Source: three-view drawing plus pictorial views. Frame: mm from the lowest corner of the part. Coordinates: 2 decimals unless noted, no trailing zeros. Write each loop counter-clockwise with the first axis right and the second up, starting at its lowest first coordinate (ties: lowest second). Pieces come first, ordered by that corner, then holes. Notation, with made-up numbers: (77.5, 53.25) - (98.5, 53.25) arc R37 ccw to (98.5, 92.25) - close; hole circle Ø9 at (39, 8). An arc over 180 degrees is marked (long way). One line per item, written item: value.
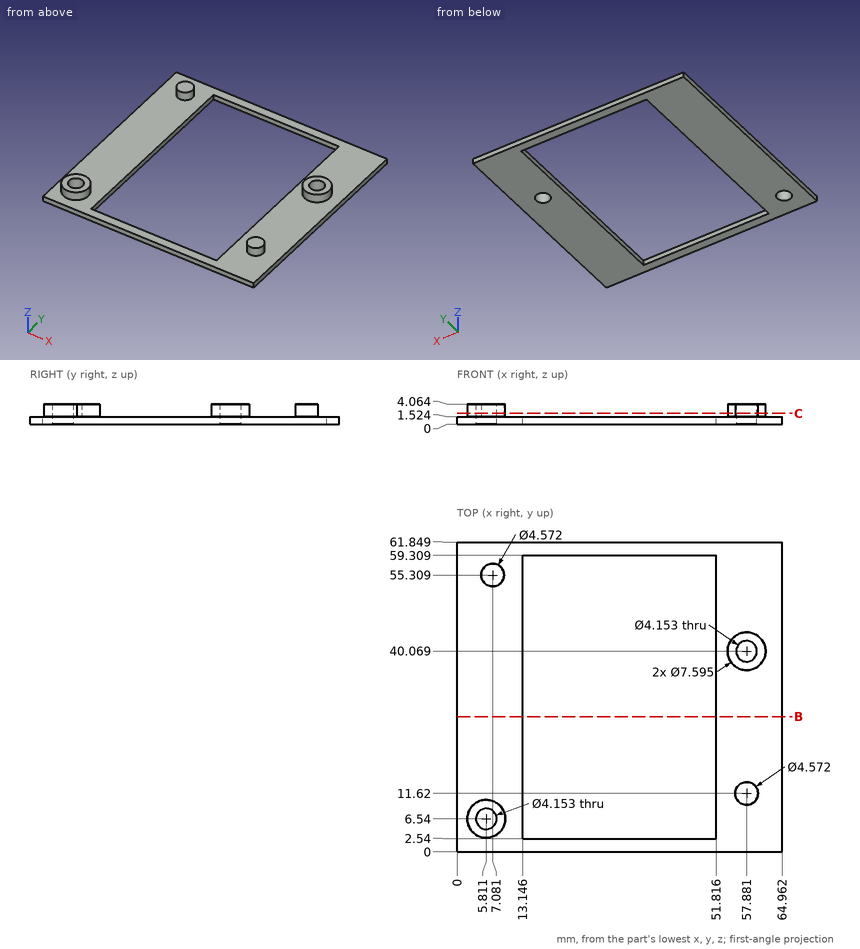
1) Section query C-C on z = 2.2. Output: boundary loops of the cut face in (x, y) (1 decimal).
Values found:
outline: circle Ø7.6 at (5.8, 6.5); circle Ø4.6 at (7.1, 55.3); circle Ø7.6 at (57.9, 40.1); circle Ø4.6 at (57.9, 11.6); hole circle Ø4.2 at (5.8, 6.5); hole circle Ø4.2 at (57.9, 40.1)
2) Contact query for a flat-ended pin moving along its axis: P1, Ø10, axis at x = 7, y = 33, coming from the +Z side. Output: stop coordinate, or through.
Values found:
P1: z = 1.52
3) Material intervals for line 1 (X direction, y = 6.5, z = 0.9) (1 decimal); line 2 (Y direction, x = 37, z = 0.3); line 3 (X direction, y = 9.5, z = 0.95) (1 decimal), sorted ascending.
Values found:
line 1: 0 to 3.7, 7.9 to 13.1, 51.8 to 65
line 2: 0 to 2.54, 59.31 to 61.85
line 3: 0 to 13.1, 51.8 to 65
4) Section query B-B on y = 27. Output: boundary loops of the cut face in (x, z) (1 decimal).
Values found:
outline: (0, 0) - (13.1, 0) - (13.1, 1.5) - (0, 1.5) - close; (51.8, 0) - (65, 0) - (65, 1.5) - (51.8, 1.5) - close
